The model under review builds one solid part; all positions refer to its coordinate system, in mm. Face numbers are marked on the shaded views. A direction names the side the tool comes from. Coordinates: 2 decimals unless noted, no trailing zeros. Write each loop counter-clockwise with the first axis right and the second up, starting at its lowest first coordinate (ties: lowest second). Pieces come first, ordered by that corner, then holes. Notation, with made-up numbers: (38.5, -13) -> (65.5, -13) arc R24 ccw to (65.5, 6) -> close; hole circle Ø6 at (6, 9.5). An arc over 180 degrees is marked (long way). Put each result on its own line as item: value. Start each with the question number.
Autodesk Inventor part; units mm, degrees
ref_plane "Work Plane1" through (21, 2, 0) normal (1, 0, 0) x (0, 0, -1)
ref_plane "Work Plane2" through (21, 2, 0) normal (1, 0, 0) x (0, 0, -1)
ref_plane "YZ Plane" through (0, 0, 0) normal (1, 0, 0) x (0, 1, 0)
sketch "Sketch1" plane through (0, 0, 0) normal (0, 0, 1) x (1, 0, 0)
  line L0 (0, 0) -> (42, 0)
  line L1 (42, 0) -> (42, 42)
  line L2 (42, 42) -> (0, 42)
  line L3 (0, 42) -> (0, 0)
  dimension "d0" = 42
  dimension "d1" = 42
extrude "Extrusion1" add sketch "Sketch1" along normal blind 47
chamfer "Chamfer1" distance 2 angle 45 4 edges at (42, 42, 23.5) (0, 42, 23.5) (42, 0, 23.5) (0, 0, 23.5)
sketch "Sketch2" plane through (0, 0, 47) normal (0, 0, 1) x (1, 0, 0)
  circle A0 centre (21, 21) radius 11
  line L0 (42, 2) -> (42, 40)
  line L1 (40, 42) -> (2, 42)
  point P0 (0, 0)
  point P1 (21, 42)
  dimension "d7" = 22
  dimension "d10" = 21
  dimension "d11" = 21
extrude "Extrusion2" add sketch "Sketch2" along normal blind 2
sketch "Sketch3" plane through (21, 21, 49) normal (0, 0, 1) x (1, 0, 0)
  circle A0 centre (0, 0) radius 2.75
  circle A1 centre (0, 0) radius 11
  point P0 (-21, -21)
  dimension "d14" = 5.5
extrude "Extrusion3" add sketch "Sketch3" along normal blind 24 from surface at -2 contours A0
sketch "Sketch4" plane through (0, 0, 47) normal (0, 0, 1) x (1, 0, 0)
  circle A0 centre (21, 21) radius 11
  line L0 (2, 0) -> (0, 2)
  line L1 (2, 0) -> (40, 0)
  line L2 (42, 2) -> (40, 0)
  line L3 (42, 2) -> (42, 40)
  line L4 (40, 42) -> (42, 40)
  line L5 (40, 42) -> (2, 42)
  line L6 (0, 40) -> (2, 42)
  line L7 (0, 40) -> (0, 2)
  circle A1 centre (21, 21) radius 2.75
  circle A2 centre (21, 21) radius 11
  circle A3 centre (21, 21) radius 2.75
  line L8 (5.5, 5.5) -> (36.5, 5.5)
  line L9 (36.5, 5.5) -> (36.5, 36.5)
  line L10 (36.5, 36.5) -> (5.5, 36.5)
  line L11 (5.5, 36.5) -> (5.5, 5.5)
  line L12 (5.5, 5.5) -> (36.5, 36.5) construction
  line L13 (36.5, 5.5) -> (5.5, 36.5) construction
  circle A4 centre (5.5, 5.5) radius 1.5
  circle A5 centre (5.5, 36.5) radius 1.5
  circle A6 centre (36.5, 36.5) radius 1.5
  circle A7 centre (36.5, 5.5) radius 1.5
  point P0 (0, 0)
  dimension "d17" = 31
  dimension "d18" = 31
  dimension "d19" = 3
extrude "Extrusion4" cut sketch "Sketch4" against normal blind 4.5 contours L11 A4 L8 | L8 A4 L11 | A7 L9 L8 | L8 L9 A7 | A5 L10 L11 | L11 L10 A5 | A6 L10 L9 | L9 L10 A6
ref_plane "Work Plane1" through (21, 2, 0) normal (1, 0, 0) x (0, 0, -1)
ref_plane "Work Plane2" through (21, 2, 0) normal (1, 0, 0) x (0, 0, -1)
properties part number "stepper motor" material "Aluminum"
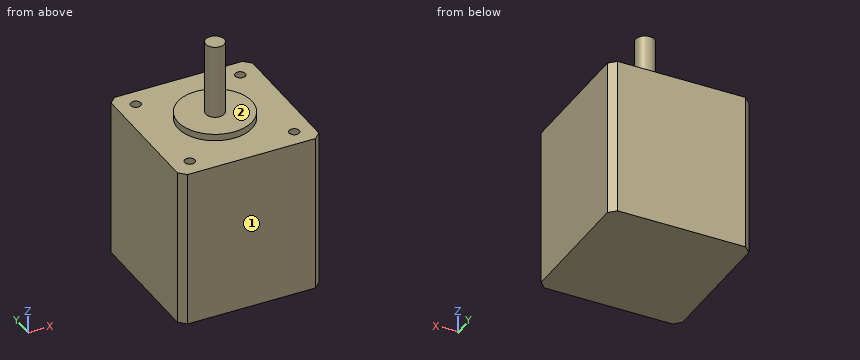
1. Consider section A-A on x = 36.5. State the section outline as (y, z) points, then the cut area to 3 significant figures.
2. Consider section D-D on x = 12.5. State the section outline as (y, z) points, then the cut area to 3 significant figures.
3. Wall thickness on line 1 (Y direction, x = 5.5, z = 45.65); line 2 (Z direction, x = 29, y = 32.5); line 3 (Y direction, x = 5, z = 45): over which ranges is each line inside the solid? List them lowest first. Write a range as from..to.
4. Consider section C-C on z = 62. State the section outline as (x, y) points, then the cut area to 3 significant figures.
5. Tool access review of the marked faces 1 and 2: name each direction out of +Z, -Z, +X, -X, +Y, -Y from which nothing blocks a thin tool from reaching the whole face with its end or side.
6. Insertion check: P1, Ø24, axis at x = 25, y = 25, coming from the +Z side; P2, Ø3.5, axis at x = 5.5, y = 36.5, coming from the +Z side; P3, Ø4, axis at x = 13.5, y = 21.5, coming from the +Z side; P4, Ø0.9, axis at x = 5, y = 36, coming from the +Z side. Each pin has a flat end and moves straight along its axis. Give the tip position at first contact, or say it passes through.
Output values:
1. outline: (0, 0) -> (42, 0) -> (42, 47) -> (38, 47) -> (38, 42.5) -> (35, 42.5) -> (35, 47) -> (7, 47) -> (7, 42.5) -> (4, 42.5) -> (4, 47) -> (0, 47) -> close
1. area: 1,950 mm^2
2. outline: (0, 0) -> (42, 0) -> (42, 47) -> (27.98, 47) -> (27.98, 49) -> (14.02, 49) -> (14.02, 47) -> (0, 47) -> close
2. area: 2,000 mm^2
3. line 1: y = 0..4, 7..35, 38..42
3. line 2: z = 0..47
3. line 3: y = 0..4.09, 6.91..35.09, 37.91..42
4. outline: circle Ø5.5 at (21, 21)
4. area: 23.8 mm^2
5. face 1: +Z, -Z, +X, -X, -Y
5. face 2: +Z
6. P1: stops at z = 71
6. P2: stops at z = 47
6. P3: stops at z = 49
6. P4: stops at z = 42.5
